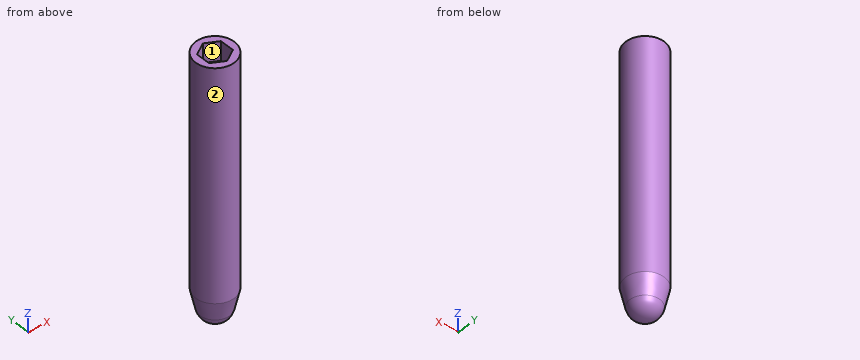
from build123d import *

# Parameters (mm, degrees)
SKETCH1_R           = 3.175
BOSS_EXTRUDE1_DEPTH = 38.1
CUT_EXTRUDE1_DEPTH  = 3.175


with BuildPart() as part:
    # Sketch1 → Boss-Extrude1 (new body)
    with BuildSketch(Plane.XY):
        Circle(SKETCH1_R)
    extrude(amount=BOSS_EXTRUDE1_DEPTH)

    # Sketch2 → Cut-Extrude1 (cut)
    with BuildSketch(Plane.XY.offset(38.1)):
        Polygon((0, 2.291358881), (-1.984375, 1.14567944), (-1.984375, -1.14567944), (0, -2.291358881), (1.984375, -1.14567944), (1.984375, 1.14567944), align=None)
    extrude(amount=-CUT_EXTRUDE1_DEPTH, mode=Mode.SUBTRACT)

    # Sketch3 → Revolve1 (revolve)
    with BuildSketch(Plane(origin=(0, 0, 0), x_dir=(1, 0, 0), z_dir=(0, 1, 0))):
        with BuildLine():
            Line((-3.175, 0), (-2.453715979, 3.222429819))
            ThreePointArc((-2.453715979, 3.222429819), (-1.567259814, 4.600861122), (0, 5.08))
            Line((0, 5.08), (0, 0))
            Line((0, 0), (-3.175, 0))
        make_face()
    revolve(axis=Axis((0, 0, -5.08), (0, 0, 1)))


solid = part.part
Work out the finished part from the listing and answer in its coordinate system (mm). Face numbers are marked on the shaded views. Coordinates: 2 decimals unless noted, no trailing zeros. Write each loop counter-clockwise with the first axis right and the second up, starting at its lowest first coordinate (ties: lowest second). Pieces come first, ordered by that corner, then holes. Notation, with made-up numbers: M 68.5,70.5 L 111.5,70.5 A11 cw 111.5,89.5 Z; hole C 51,47.5 d3. An arc over 180 degrees is marked long. Answer as CSV lines item,"result". Start each with the question number.
Item 1: Determine the mould class of the marked faces 1 and 2 for opening direction Y: released by +Y, released by -Y, zero draft, split by the parting line, or undercut.
Item 2: Section A-A on z = 10.5 is taken. Write down the section's boundary in (x, y) (3 decimals), and give its area (3 significant figures).
Item 3: Consider L1, parallel to Z at x = -0.5, y = 0.5 (3 decimals); L2, parallel to X at y = 0.75, z = 6. Determine where each line is inside the solid, lowest interval first.
Item 4: Flat-ended cylindrical pins translate along their axes: P1, Ø1.5, axis at x = 1.5, z = 4, coming from the -Y side; P2, Ø2, axis at y = -2, z = 0, coming from the +X side; P3, Ø1.2, axis at x = -0.5, y = -0.5, coming from the +Z side (3 decimals). Find the tip coordinate at first contact, or state that the pin passes through.
Checks:
1,face 1,"undercut"
1,face 2,"split by the parting line"
2,outline,"C 0,0 d6.35"
2,area,"31.7 mm²"
3,L1,"z = -5.013 to 34.925"
3,L2,"x = -3.09 to 3.09"
4,P1,"stops at y = -3.09"
4,P2,"stops at x = 3.01"
4,P3,"stops at z = 34.925"
